from build123d import *

# Parameters (mm, degrees)
SKETCH1_R                   = 27.5
BOSS_EXTRUDE1_DEPTH         = 23
M12X1_75_TAPPED_HOLE1_D     = 10.2
M12X1_75_TAPPED_HOLE1_DEPTH = 21
M12X1_75_TAPPED_HOLE1_TIP   = 3.064389157
SKETCH9_R                   = 11
CUT_EXTRUDE1_DEPTH          = 10
M8X1_25_TAPPED_HOLE1_D      = 6.8
M8X1_25_TAPPED_HOLE1_DEPTH  = 16
M8X1_25_TAPPED_HOLE1_TIP    = 2.042926105


with BuildPart() as part:
    # Sketch1 → Boss-Extrude1 (new body)
    with BuildSketch(Plane(origin=(0, 0, 0), x_dir=(1, 0, 0), z_dir=(0, 1, 0))):
        Circle(SKETCH1_R)
    extrude(amount=BOSS_EXTRUDE1_DEPTH)

    # Sketch3 → Cut-Revolve1 (revolve, cut)
    with BuildSketch(Plane(origin=(0, 0, 0), x_dir=(0, 0, -1), z_dir=(1, 0, 0))):
        Polygon((-27.5, 16), (-5.5, 23), (-27.5, 23), align=None)
    revolve(axis=Axis((0, 0, 0), (0, 1, 0)), mode=Mode.SUBTRACT)

    # M12x1.75 Tapped Hole1
    with Locations(Plane.ZX.offset(23)):
        with Locations((0, 0)):
            Hole(M12X1_75_TAPPED_HOLE1_D / 2, depth=M12X1_75_TAPPED_HOLE1_DEPTH)
            with Locations((0, 0, -(M12X1_75_TAPPED_HOLE1_DEPTH + M12X1_75_TAPPED_HOLE1_TIP / 2))):  # 118° drill point
                Cone(0, M12X1_75_TAPPED_HOLE1_D / 2, M12X1_75_TAPPED_HOLE1_TIP, mode=Mode.SUBTRACT)

    # Sketch9 → Cut-Extrude1 (cut)
    with BuildSketch(Plane.XZ):
        Circle(SKETCH9_R)
    extrude(amount=-CUT_EXTRUDE1_DEPTH, mode=Mode.SUBTRACT)

    # M8x1.25 Tapped Hole1
    with Locations(Plane(origin=(0, 0, 20), x_dir=(0, 0, -1), z_dir=(0, -1, 0))):
        with Locations((0, 0), (20, 20), (40, 0), (20, -20)):
            Hole(M8X1_25_TAPPED_HOLE1_D / 2, depth=M8X1_25_TAPPED_HOLE1_DEPTH)
            with Locations((0, 0, -(M8X1_25_TAPPED_HOLE1_DEPTH + M8X1_25_TAPPED_HOLE1_TIP / 2))):  # 118° drill point
                Cone(0, M8X1_25_TAPPED_HOLE1_D / 2, M8X1_25_TAPPED_HOLE1_TIP, mode=Mode.SUBTRACT)


solid = part.part
For this review, take the finished solid that the model builds, in its own axes (mm). A direction names the side the tool comes from. Round coordinates to 2 decimals unless told otherwise and drop trailing zeros. Loops run counter-clockwise (first coordinate to the right, second up) from the corner with the lowest first, then second, coordinate; pieces in that order, holes last. Notation, with made-up numbers: (-14, 27.5) - (2, 27.5) arc R17 cw to (2, 46.5) - close; hole circle Ø4 at (52, -40). An arc over 180 degrees is marked (long way). Use one line per item in the form item = value.
Item 1: Consider section A-A on y = 9. Write out the cut boundary in (x, z).
Answers:
outline = circle Ø55 at (0, 0); hole circle Ø6.8 at (-20, 0); hole circle Ø22 at (0, 0); hole circle Ø6.8 at (0, -20); hole circle Ø6.8 at (0, 20); hole circle Ø6.8 at (20, 0)
Item 2: Consider section B-B on y = 17.25. Write out the cut boundary in (x, z).
Answers:
outline = circle Ø47.14 at (0, 0); hole circle Ø2.64 at (-20, 0); hole circle Ø10.2 at (0, 0); hole circle Ø2.64 at (0, -20); hole circle Ø2.64 at (0, 20); hole circle Ø2.64 at (20, 0)
Item 3: Mouldability with a two-part tool opening along Z and no side actions: class faces 3 (the conical face through (6.51, 22.66, -0.86)), 4 (the flat face through (0, 0, 12)), 5 (the cylindrical face through (16.68, 8.11, -0.74)) as +Z half, -Z half, draft (parallel to the pull), parting line (faces both ways), or undercut.
Answers:
face_3 = parting line
face_4 = draft
face_5 = undercut
Item 4: Tool access review of faces 1 (the cylindrical face through (-1.3, 8.11, -16.86)), 2 (the cylindrical face through (26.23, 7.89, -8.26)): name each direction out of +Z, -Z, +X, -X, +Y, -Y from which nothing blocks a thin tool from reaching the whole face with its end or side.
Answers:
face_1 = -Y
face_2 = +Y, -Y
Item 5: For line 1 (X direction, y = 13.25, z = 0); line 2 (Z direction, x = 0, y = 7); line 3 (X direction, y = 3.5, z = -2.5), list the stretches that pass through material, from the lowest coordinate up.
Answers:
line_1 = -27.5 to -23.4, -16.6 to -5.1, 5.1 to 16.6, 23.4 to 27.5
line_2 = -27.5 to -23.4, -16.6 to -11, 11 to 16.6, 23.4 to 27.5
line_3 = -27.39 to -22.3, -17.7 to -10.71, 10.71 to 17.7, 22.3 to 27.39
Item 6: Clearance check with flat-ended pins moving along their axes: P1, Ø9, axis at x = 20, z = 0, coming from the +Y side; P2, Ø10, axis at y = 6.5, z = -20, coming from the -X side; P3, Ø2, axis at y = 16, z = -10, coming from the +X side. State where each tip first meets the part, or that it passes through.
Answers:
P1 = 19.82
P2 = -23.05
P3 = 25.99
